Read the model definition and answer for the solid it produces. Units are mm, in the model's axes. A direction names the side the tool comes from. Coordinates: 2 decimals unless noted, no trailing zeros. Write each loop counter-clockwise with the first axis right and the second up, starting at its lowest first coordinate (ties: lowest second). Pieces come first, ordered by that corner, then holes. Notation, with made-up numbers: (-13.75, 35) -> (29.25, 35) arc R7 cw to (29.25, 45) -> close; hole circle Ø3 at (39.25, 58). An arc over 180 degrees is marked (long way). Answer in a Markdown table with one row per item. Add a question column.
Item 1: Given pin 1 Ø6 at (y, z) = (20.5, 34) entering from -X; pin 2 Ø10 at (x, y) = (0.5, 16) entering from +Z; pin 3 Ø12 at (x, y) = (-10.5, -17.5) entering from -Z, each flat-ended and moving along its own axis, determine where each tip first touches the part or whether it passes through.
Item 2: For a pull along Y with two mould halves and no side action, classify faces 4 (the face through (-1.08, -4.88, 154.86)), 5 (the face through (9, 25, 82)), 6 (the face through (0, 0, 0)) as +Y half, -Y half, draft (parallel to the pull), parting line (faces both ways), or undercut.
Item 3: Section A-A on y = -13 is taken. Write down the section's boundary in (x, z).
Item 4: Section C-C on z = 118 is taken. Write down the section's boundary in (x, y).
Item 5: Which of the six approach directions +Z, -Z, +X, -X, +Y, -Y give full straight-line access (tool end or side, diameter ignored) to faces 1 (the face through (0, 0, 165)), 2 (the face through (9, -25, 82)), 3 (the face through (-1.08, -4.88, 9.86))?
Item 6: Section B-B on x = 17 is taken. Write down the section's boundary in (y, z).
Item 7: Straight lines are drawn through the part: line 1 (Z direction, x = -4, y = -23.5); line 2 (Z direction, x = 0, y = 27); line 3 (X direction, y = -28, z = 82). For each, find the intervals that lie inside material, in ascending order. Write a range as from..to.
Item 8: Section D-D on x = 0 is taken. Write down the section's boundary in (y, z).
```python
from build123d import *

# Parameters (mm, degrees)
SKETCH_1_R          = 5
EXTRUDE_1_DEPTH     = 20
SKETCH_2_W          = 40
SKETCH_2_H          = 60
EXTRUDE_2_DEPTH     = 5
SKETCH_3_W          = 40
SKETCH_3_H          = 5
EXTRUDE_3_DEPTH     = 115
SKETCH_4_W          = 40
SKETCH_4_H          = 60
EXTRUDE_4_DEPTH     = 5
SKETCH_5_R          = 5
EXTRUDE_5_DEPTH     = 20
SKETCH_6_R          = 5
CUT_EXTRUDE_1_DEPTH = 241


with BuildPart() as part:
    # Эскиз1 → Бобышка-Вытянуть1 (new body)
    with BuildSketch(Plane.XY):
        Circle(SKETCH_1_R)
    extrude(amount=EXTRUDE_1_DEPTH)

    # Эскиз2 → Бобышка-Вытянуть2 (add)
    with BuildSketch(Plane.XY.offset(20)):
        Rectangle(SKETCH_2_W, SKETCH_2_H)
    extrude(amount=EXTRUDE_2_DEPTH)

    # Эскиз3 → Бобышка-Вытянуть3 (add)
    with BuildSketch(Plane.XY.offset(25)):
        with Locations((0, 27.5)):
            Rectangle(SKETCH_3_W, SKETCH_3_H)
        with Locations((0, -27.5)):
            Rectangle(SKETCH_3_W, SKETCH_3_H)
    extrude(amount=EXTRUDE_3_DEPTH)

    # Эскиз4 → Бобышка-Вытянуть4 (add)
    with BuildSketch(Plane.XY.offset(140)):
        Rectangle(SKETCH_4_W, SKETCH_4_H)
    extrude(amount=EXTRUDE_4_DEPTH)

    # Эскиз5 → Бобышка-Вытянуть5 (add)
    with BuildSketch(Plane.XY.offset(145)):
        Circle(SKETCH_5_R)
    extrude(amount=EXTRUDE_5_DEPTH)

    # Эскиз6 → Вырез-Вытянуть1 (cut)
    with BuildSketch(Plane(origin=(0, 30, 0), x_dir=(1, 0, 0), z_dir=(0, 1, 0))):
        with Locations(Location((0, -82.5, 0), (0, 0, 180))):
            Circle(SKETCH_6_R)
    extrude(amount=-CUT_EXTRUDE_1_DEPTH, mode=Mode.SUBTRACT)


solid = part.part
```
Results below:
| question | item | result |
|---|---|---|
| 1 | pin 1 | passes through |
| 1 | pin 2 | stops at z = 145 |
| 1 | pin 3 | stops at z = 20 |
| 2 | face 4 | parting line |
| 2 | face 5 | undercut |
| 2 | face 6 | draft |
| 3 | outline | (-20, 20) -> (20, 20) -> (20, 25) -> (-20, 25) -> close; (-20, 140) -> (20, 140) -> (20, 145) -> (-20, 145) -> close |
| 4 | outline | (-20, -30) -> (20, -30) -> (20, -25) -> (-20, -25) -> close; (-20, 25) -> (20, 25) -> (20, 30) -> (-20, 30) -> close |
| 5 | face 1 | +Z, +X, -X, +Y, -Y |
| 5 | face 2 | +X, -X |
| 5 | face 3 | -Z |
| 6 | outline | (-30, 20) -> (30, 20) -> (30, 145) -> (-30, 145) -> close; hole (-25, 25) -> (25, 25) -> (25, 140) -> (-25, 140) -> close |
| 7 | line 1 | z = 20..25, 140..145 |
| 7 | line 2 | z = 20..77.5, 87.5..145 |
| 7 | line 3 | x = -20..-4.97, 4.97..20 |
| 8 | outline | (-30, 20) -> (-5, 20) -> (-5, 0) -> (5, 0) -> (5, 20) -> (30, 20) -> (30, 77.5) -> (25, 77.5) -> (25, 25) -> (-25, 25) -> (-25, 77.5) -> (-30, 77.5) -> close; (-30, 87.5) -> (-25, 87.5) -> (-25, 140) -> (25, 140) -> (25, 87.5) -> (30, 87.5) -> (30, 145) -> (5, 145) -> (5, 165) -> (-5, 165) -> (-5, 145) -> (-30, 145) -> close |
